Model file for the job. Use its own axes, mm. A direction names the side the tool comes from. Coordinates: 2 decimals unless noted, no trailing zeros. Order: outer loops, then holes, each group sorted by start corner. A loop starts at its lowest first (then second) coordinate and runs counter-clockwise, first axis right, second up. Notation, with made-up numbers: M -11,80 L -7,80 A19 ccw -7,88 Z; hole C 42,65.5 d11. An arc over 180 degrees is marked long. Return JSON: item names as keys, results as strings.
```python
from build123d import *

# Parameters (mm, degrees)
F0_R     = 29
F1_DEPTH = 8


with BuildPart() as f1:
    # F0 (on Front) → F1 (new body)
    with BuildSketch(Plane.XZ):
        Circle(F0_R)
        with BuildLine():
            ThreePointArc((0.5, 24.9949994999), (17.6776695297, 17.6776695297), (24.9949994999, 0.5))
            ThreePointArc((24.9949994999, 0.5), (24.9987498437, 0.2500125022), (25, 0))
            ThreePointArc((25, 0), (24.9987498437, -0.2500125022), (24.9949994999, -0.5))
            ThreePointArc((24.9949994999, -0.5), (17.6776695297, -17.6776695297), (0.5, -24.9949994999))
            ThreePointArc((0.5, -24.9949994999), (0, -25), (-0.5, -24.9949994999))
            ThreePointArc((-0.5, -24.9949994999), (-17.6776695297, -17.6776695297), (-24.9949994999, -0.5))
            ThreePointArc((-24.9949994999, -0.5), (-25, 0), (-24.9949994999, 0.5))
            ThreePointArc((-24.9949994999, 0.5), (-17.6776695297, 17.6776695297), (-0.5, 24.9949994999))
            ThreePointArc((-0.5, 24.9949994999), (0, 25), (0.5, 24.9949994999))
        make_face(mode=Mode.SUBTRACT)
        with BuildLine():
            ThreePointArc((1.9364916731, 0.5), (1.9840593925, 0.252008585), (2, 0))
            ThreePointArc((2, 0), (1.9840593925, -0.252008585), (1.9364916731, -0.5))
            Line((1.9364916731, -0.5), (2.9580398915, -0.5))
            ThreePointArc((2.9580398915, -0.5), (2.9894915684, -0.2508787808), (3, 0))
            ThreePointArc((3, 0), (2.9894915684, 0.2508787808), (2.9580398915, 0.5))
            Line((2.9580398915, 0.5), (1.9364916731, 0.5))
        make_face()
        with BuildLine():
            ThreePointArc((1.5931753199, 1.2090460702), (1.8000899569, 0.8715940265), (1.9364916731, 0.5))
            Line((1.9364916731, 0.5), (2.9580398915, 0.5))
            ThreePointArc((2.9580398915, 0.5), (2.7533824356, 1.1911696619), (2.3897629799, 1.8135691053))
            Line((2.3897629799, 1.8135691053), (1.5931753199, 1.2090460702))
        make_face()
        with BuildLine():
            Line((2.9580398915, -0.5), (1.9364916731, -0.5))
            ThreePointArc((1.9364916731, -0.5), (1.4142135624, -1.4142135624), (0.5, -1.9364916731))
            Line((0.5, -1.9364916731), (0.5, -2.9580398915))
            ThreePointArc((0.5, -2.9580398915), (2.1213203436, -2.1213203436), (2.9580398915, -0.5))
        make_face()
        with BuildLine():
            Line((24.9949994999, 0.5), (2.9580398915, 0.5))
            ThreePointArc((2.9580398915, 0.5), (2.9894915684, 0.2508787808), (3, 0))
            ThreePointArc((3, 0), (2.9894915684, -0.2508787808), (2.9580398915, -0.5))
            Line((2.9580398915, -0.5), (24.9949994999, -0.5))
            ThreePointArc((24.9949994999, -0.5), (24.9987498437, -0.2500125022), (25, 0))
            ThreePointArc((25, 0), (24.9987498437, 0.2500125022), (24.9949994999, 0.5))
        make_face()
        with BuildLine():
            Line((0.5, -2.9580398915), (0.5, -1.9364916731))
            ThreePointArc((0.5, -1.9364916731), (0, -2), (-0.5, -1.9364916731))
            Line((-0.5, -1.9364916731), (-0.5, -2.9580398915))
            ThreePointArc((-0.5, -2.9580398915), (0, -3), (0.5, -2.9580398915))
        make_face()
        with BuildLine():
            ThreePointArc((0.5, 1.9364916731), (0.7937447605, 1.8357476012), (1.068353257, 1.6907457876))
            Line((1.068353257, 1.6907457876), (1.6025298855, 2.5361186814))
            ThreePointArc((1.6025298855, 2.5361186814), (1.0722230909, 2.8018453996), (0.5, 2.9580398915))
            Line((0.5, 2.9580398915), (0.5, 1.9364916731))
        make_face()
        with BuildLine():
            Line((-0.5, -2.9580398915), (-0.5, -1.9364916731))
            ThreePointArc((-0.5, -1.9364916731), (-1.4142135624, -1.4142135624), (-1.9364916731, -0.5))
            Line((-1.9364916731, -0.5), (-2.9580398915, -0.5))
            ThreePointArc((-2.9580398915, -0.5), (-2.1213203436, -2.1213203436), (-0.5, -2.9580398915))
        make_face()
        with BuildLine():
            Line((0.5, -24.9949994999), (0.5, -2.9580398915))
            ThreePointArc((0.5, -2.9580398915), (0, -3), (-0.5, -2.9580398915))
            Line((-0.5, -2.9580398915), (-0.5, -24.9949994999))
            ThreePointArc((-0.5, -24.9949994999), (0, -25), (0.5, -24.9949994999))
        make_face()
        with BuildLine():
            ThreePointArc((-0.5, 1.9364916731), (0, 2), (0.5, 1.9364916731))
            Line((0.5, 1.9364916731), (0.5, 2.9580398915))
            ThreePointArc((0.5, 2.9580398915), (0, 3), (-0.5, 2.9580398915))
            Line((-0.5, 2.9580398915), (-0.5, 1.9364916731))
        make_face()
        with BuildLine():
            Line((0.5, 2.9580398915), (0.5, 24.9949994999))
            ThreePointArc((0.5, 24.9949994999), (0, 25), (-0.5, 24.9949994999))
            Line((-0.5, 24.9949994999), (-0.5, 2.9580398915))
            ThreePointArc((-0.5, 2.9580398915), (0, 3), (0.5, 2.9580398915))
        make_face()
        with BuildLine():
            Line((-2.9580398915, -0.5), (-1.9364916731, -0.5))
            ThreePointArc((-1.9364916731, -0.5), (-2, 0), (-1.9364916731, 0.5))
            Line((-1.9364916731, 0.5), (-2.9580398915, 0.5))
            ThreePointArc((-2.9580398915, 0.5), (-3, 0), (-2.9580398915, -0.5))
        make_face()
        with BuildLine():
            ThreePointArc((-1.9364916731, 0.5), (-1.4142135624, 1.4142135624), (-0.5, 1.9364916731))
            Line((-0.5, 1.9364916731), (-0.5, 2.9580398915))
            ThreePointArc((-0.5, 2.9580398915), (-2.1213203436, 2.1213203436), (-2.9580398915, 0.5))
            Line((-2.9580398915, 0.5), (-1.9364916731, 0.5))
        make_face()
        with BuildLine():
            Line((-24.9949994999, -0.5), (-2.9580398915, -0.5))
            ThreePointArc((-2.9580398915, -0.5), (-3, 0), (-2.9580398915, 0.5))
            Line((-2.9580398915, 0.5), (-24.9949994999, 0.5))
            ThreePointArc((-24.9949994999, 0.5), (-25, 0), (-24.9949994999, -0.5))
        make_face()
    extrude(amount=F1_DEPTH)


solid = f1.part
```
Item 1: Saw through at C-C (y = -3.5). Write the cut outline in (x, z) (1 decimal).
Check result:
{"outline": "C 0,0 d58; hole M -25,-0.5 A25 ccw -0.5,-25 L -0.5,-3 A3 cw -3,-0.5 Z; hole M -25,0.5 L -3,0.5 A3 cw -0.5,3 L -0.5,25 A25 ccw Z; hole M 0.5,-25 A25 ccw 25,-0.5 L 3,-0.5 A3 cw 0.5,-3 Z; hole M 0.5,3 A3 cw 1.6,2.5 L 1.1,1.7 A2 ccw long 1.6,1.2 L 2.4,1.8 A3 cw 3,0.5 L 25,0.5 A25 ccw 0.5,25 Z"}
Item 2: Saw through at B-B (z = 22). Write the cut outline in (x, y), and give its area (3 significant figures).
Check result:
{"outline": "M -18.89,-8 L -11.87,-8 L -11.87,0 L -18.89,0 Z; M -0.5,-8 L 0.5,-8 L 0.5,0 L -0.5,0 Z; M 11.87,-8 L 18.89,-8 L 18.89,0 L 11.87,0 Z", "area": "120 mm2"}
Item 3: Pull direction Z, two halves, no side cores. Call faces 3 (the cylindrical face through (13.38, -3.94, -25.73)), 4 (the flat face through (-14, -4, -0.5)), 5 (the cylindrical face through (-17.866, -3.944, 17.487)), 6 (the flat face through (6, -8, 0)): +Z half, -Z half, draft (parallel to the pull), parting line (faces both ways), or undercut.
Check result:
{"face 3": "parting line", "face 4": "undercut", "face 5": "undercut", "face 6": "draft"}
Item 4: Drop flat-ended pins along their axis: pin 1 Ø4 at (y, z) = (-5, -14.5) entering from -X; pin 2 Ø1 at (x, y) = (10, -5) entering from +Z; pin 3 Ø1.5 at (y, z) = (-4.5, 20) entering from +X. Give the stop position or say it passes through.
Check result:
{"pin 1": "stops at x = -26.17", "pin 2": "stops at z = 27.4", "pin 3": "stops at x = 21.69"}
Item 5: Wall check: line 1 (Z direction, x = 15.5, y = -4); line 2 (X direction, y = -5.75, z = -13); line 3 (Z direction, x = 12.5, y = -7.25). Give the ranges that are in metal, low to high.
Check result:
{"line 1": "z = -24.51 to -19.62, -0.5 to 0.5, 19.62 to 24.51", "line 2": "x = -25.92 to -21.35, -0.5 to 0.5, 21.35 to 25.92", "line 3": "z = -26.17 to -21.65, -0.5 to 0.5, 21.65 to 26.17"}
Item 6: 3-axis set-ups, long thin cutter, end or side, ignore diameter. For faces 1 (the flat face through (0.5, -4, -14)), 2 (the flat face through (6, 0, 0)): which of +Z, -Z, +X, -X, +Y, -Y reach the whole face in a straight line?
Check result:
{"face 1": "+Y, -Y", "face 2": "+Z, -Z, +X, -X, +Y"}
Item 7: Saw through at A-A (x = 20). Write the cut outline in (y, z).
Check result:
{"outline": "M -8,-21 L 0,-21 L 0,-15 L -8,-15 Z; M -8,-0.5 L 0,-0.5 L 0,0.5 L -8,0.5 Z; M -8,15 L 0,15 L 0,21 L -8,21 Z"}
